Read the model definition and answer for the solid it produces. Units are mm, in the model's axes. A direction names the side the tool comes from. Coordinates: 2 decimals unless noted, no trailing zeros. Write each loop counter-clockwise with the first axis right and the second up, starting at its lowest first coordinate (ties: lowest second). Pieces come first, ordered by that corner, then holes.
(1) The part is cut by section C-C, the plane y = 4. Determine the outline of the cut face in (x, z), and give its area (3 significant figures).
(2) The part is cut by section B-B, the plane y = 2.05. Determine the outline of the cut face in (x, z), and give its area (3 significant figures).
(3) Determine the mould class of faces 3 (the cylindrical face through (-25, 1, 0)), 4 (the cylindrical face through (-18.735, 1.479, 0.806)), 5 (the flat face through (0, 0, 0)) for opening direction X: pulls with the +X half, pulls with the -X half, needs draft (parallel to the pull), parting line crosses it, or undercut.
(4) The part is cut by section D-D, the plane z = 0. State how many separate pieces and enclosed holes the cut face has, and give its area (3 significant figures).
(5) Straight lines are drawn through the part: line 1 along X through (y, z) = (0.9, 0); line 2 along Z through (x, y) = (10, 1.3); line 3 along X through (y, z) = (5.15, 0). For each, find the intervals that lie inside material, in ascending order.
(6) Which of the six approach directions +Z, -Z, +X, -X, +Y, -Y give full straight-line access (tool end or side, diameter ignored) to faces 1 (the flat face through (0, 3, 0)), 2 (the flat face through (0, 1, -5))?
(7) Given pin 1 (5 mm diameter, centred on x = 10, z = 0, fed in from +Y); pin 2 (6 mm diameter, centred on x = 8, z = -0.5, fed in from -Y); pin 3 (2.5 mm diameter, centred on x = -20, z = 0, fed in from +Y), each flat-ended and moving along its own axis, determine where each tip first touches the part or whether it passes through.
(8) The part is cut by section A-A, the plane x = -10. Determine the outline of the cut face in (y, z), and give its area (3 significant figures).
```python
from build123d import *

# Parameters (mm, degrees)
SKETCH1_W           = 50
SKETCH1_H           = 10
SKETCH1_R           = 1.5
BOSS_EXTRUDE1_DEPTH = 3
FILLET2_RADIUS      = 5
FILLET2_LENGTH      = 3
FILLET3_RADIUS      = 5
FILLET3_LENGTH      = 3
SKETCH2_R           = 3.8
SKETCH2_R_2         = 2.8
BOSS_EXTRUDE2_DEPTH = 3
FILLET4_R           = 0.2


with BuildPart() as part:
    # Sketch1 → Boss-Extrude1 (new body)
    with BuildSketch(Plane(origin=(0, 0, 0), x_dir=(1, 0, 0), z_dir=(0, 1, 0))):
        Rectangle(SKETCH1_W, SKETCH1_H)
        with Locations(Location((-20, 0, 0), (0, 0, 270))):
            Circle(SKETCH1_R, mode=Mode.SUBTRACT)
        with Locations(Location((-10, 0, 0), (0, 0, 270))):
            Circle(SKETCH1_R, mode=Mode.SUBTRACT)
        with Locations(Location((10, 0, 0), (0, 0, 90))):
            Circle(SKETCH1_R, mode=Mode.SUBTRACT)
        with Locations(Location((20, 0, 0), (0, 0, 90))):
            Circle(SKETCH1_R, mode=Mode.SUBTRACT)
    extrude(amount=BOSS_EXTRUDE1_DEPTH)

    # Fillet2: full round fillet: the end face becomes a half cylinder, R = half its width
    fillet2_face = Plane((-25, 1.5, 0), x_dir=(0, -1, 0), z_dir=(-1, 0, 0))  # on the end face: x along it, z out of the body
    fillet2_slab = fillet2_face.offset(-FILLET2_RADIUS / 2) * Box(FILLET2_LENGTH, 2 * FILLET2_RADIUS, FILLET2_RADIUS, mode=Mode.PRIVATE)  # the body's end, R deep
    fillet2_round = Plane((-20, 1.5, 0), x_dir=(-1, 0, 0), z_dir=(0, -1, 0)) * Cylinder(FILLET2_RADIUS, FILLET2_LENGTH, mode=Mode.PRIVATE)  # its axis R under the face
    add(fillet2_slab - fillet2_round, mode=Mode.SUBTRACT)

    # Fillet3: full round fillet: the end face becomes a half cylinder, R = half its width
    fillet3_face = Plane((25, 1.5, 0), x_dir=(0, 1, 0), z_dir=(1, 0, 0))  # on the end face: x along it, z out of the body
    fillet3_slab = fillet3_face.offset(-FILLET3_RADIUS / 2) * Box(FILLET3_LENGTH, 2 * FILLET3_RADIUS, FILLET3_RADIUS, mode=Mode.PRIVATE)  # the body's end, R deep
    fillet3_round = Plane((20, 1.5, 0), x_dir=(1, 0, 0), z_dir=(0, 1, 0)) * Cylinder(FILLET3_RADIUS, FILLET3_LENGTH, mode=Mode.PRIVATE)  # its axis R under the face
    add(fillet3_slab - fillet3_round, mode=Mode.SUBTRACT)

    # Sketch2 → Boss-Extrude2 (add)
    with BuildSketch(Plane(origin=(0, 3, 0), x_dir=(1, 0, 0), z_dir=(0, 1, 0))):
        with Locations(Location((0, 0, 0), (0, 0, 270))):
            Circle(SKETCH2_R)
        with Locations(Location((0, 0, 0), (0, 0, 270))):
            Circle(SKETCH2_R_2, mode=Mode.SUBTRACT)
    extrude(amount=BOSS_EXTRUDE2_DEPTH)

    # Fillet4
    fillet4_edges = [part.edges().sort_by_distance(p)[0] for p in [
        (0, 0, 5),
        (0, 3, 5),
        (-25, 0, 0),
        (-25, 3, 0),
        (0, 0, -5),
        (0, 3, -5),
        (25, 0, 0),
        (25, 3, 0),
        (0, 6, -3.8),
        (0, 3, -3.8),
        (0, 6, -2.8),
    ]]
    fillet(fillet4_edges, radius=FILLET4_R)


solid = part.part
```
Computed:
1. outline: circle Ø7.6 at (0, 0); hole circle Ø5.6 at (0, 0)
1. area: 20.7 mm2
2. outline: (-20, -5) - (20, -5) arc R5 ccw to (20, 5) - (-20, 5) arc R5 ccw to start; hole circle Ø3 at (-20, 0); hole circle Ø3 at (-10, 0); hole circle Ø3 at (10, 0); hole circle Ø3 at (20, 0)
2. area: 450 mm2
3. face 3: pulls with the -X half
3. face 4: undercut
3. face 5: needs draft
4. separate pieces: 5
4. enclosed holes: 0
4. area: 120 mm2
5. line 1: x = -25 to -21.5, -18.5 to -11.5, -8.5 to 8.5, 11.5 to 18.5, 21.5 to 25
5. line 2: z = -5 to -1.5, 1.5 to 5
5. line 3: x = -3.8 to -2.8, 2.8 to 3.8
6. face 1: +Y
6. face 2: -Z, +X, -X, +Y, -Y
7. pin 1: stops at y = 3
7. pin 2: stops at y = 0
7. pin 3: passes through
8. outline: (0, -4.8) arc R0.2 ccw to (0.2, -5) - (2.8, -5) arc R0.2 ccw to (3, -4.8) - (3, -1.5) - (0, -1.5) - close; (0, 1.5) - (3, 1.5) - (3, 4.8) arc R0.2 ccw to (2.8, 5) - (0.2, 5) arc R0.2 ccw to (0, 4.8) - close
8. area: 21.0 mm2
